from build123d import *

# Parameters (mm, degrees)
MAIN_FACE_EXTRUDE_DEPTH              = 7.4
MAIN_WALLS_EXTRUDE_DEPTH             = 35
MAIN_WALLS_LOWER_CHAMFER_SIZE        = 1
MAIN_WALLS_ENTRY_CHAMFER_SIZE        = 1
SKETCH4_W                            = 3
SKETCH4_H                            = 40.5
SERVO_MOUNT_CUT_DEPTH                = 35
SERVO_MOUNT_HOLES_REACH              = 72.134
SKETCH5_R                            = 2.25
MOUNT_DOVETAIL_DEPTH                 = 61.8
MOUNT_DOVETAIL_CHAMFER_SIZE          = 8
SKETCH9_W                            = 27.3
SKETCH9_H                            = 68.845299462
DOVETAIL_OFFSET_CUT_DEPTH            = 5
SKETCH10_R                           = 2.05
MOUNT_SCREW_HOLE_DEPTH               = 72.175838597
SKETCH11_R                           = 3.5
MOUNT_SCREW_COUNTERSINK_DEPTH        = 3
MOUNT_SCREW_COUNTERSINK_CHAMFER_SIZE = 1
GEAR_CUT_DEPTH                       = 68.031634323
GEAR_ENTRY_CHAMFER_SIZE              = 3


with BuildPart() as part:
    # Sketch1 → Main Face Extrude (new body)
    with BuildSketch(Plane(origin=(0, 0, 0), x_dir=(1, 0, 0), z_dir=(0, 1, 0))):
        Polygon((-20, 35), (7.542640687, 35), (20, 22.542640687), (20, -26.542640687), (7.542640687, -39), (-20, -39), align=None)
    extrude(amount=MAIN_FACE_EXTRUDE_DEPTH)

    # Sketch3 → Main Walls Extrude (add)
    with BuildSketch(Plane(origin=(0, 7.4, 0), x_dir=(1, 0, 0), z_dir=(0, 1, 0))):
        Polygon((-20, 35), (-20, -39), (7.542640687, -39), (20, -26.542640687), (20, 22.542640687), (7.542640687, 35), align=None)
        Polygon((-17, 32), (-17, -36), (6.3, -36), (17, -25.3), (17, 21.3), (6.3, 32), align=None, mode=Mode.SUBTRACT)
    extrude(amount=MAIN_WALLS_EXTRUDE_DEPTH)

    # Main Walls Lower Chamfer
    main_walls_lower_chamfer_edges = [part.edges().sort_by_distance(p)[0] for p in [
        (-5.35, 7.4, -32),
        (-5.35, 7.4, 36),
        (11.65, 7.4, 30.65),
        (17, 7.4, 2),
        (11.65, 7.4, -26.65),
    ]]
    chamfer(main_walls_lower_chamfer_edges, length=MAIN_WALLS_LOWER_CHAMFER_SIZE)

    # Main Walls Entry Chamfer
    main_walls_entry_chamfer_edges = [part.edges().sort_by_distance(p)[0] for p in [
        (-5.35, 42.4, -32),
        (-17, 42.4, 2),
        (-5.35, 42.4, 36),
        (11.65, 42.4, 30.65),
        (17, 42.4, 2),
        (11.65, 42.4, -26.65),
    ]]
    chamfer(main_walls_entry_chamfer_edges, length=MAIN_WALLS_ENTRY_CHAMFER_SIZE)

    # Sketch4 → Servo Mount Cut (cut)
    with BuildSketch(Plane(origin=(0, 42.4, 0), x_dir=(1, 0, 0), z_dir=(0, 1, 0))):
        with Locations((-18.5, -3.45)):
            Rectangle(SKETCH4_W, SKETCH4_H)
    extrude(amount=-SERVO_MOUNT_CUT_DEPTH, mode=Mode.SUBTRACT)

    # Sketch5 → Servo Mount Holes (cut, up to next)
    with BuildSketch(Plane.ZY.offset(20), mode=Mode.PRIVATE) as servo_mount_holes_sk1:
        with Locations((-21.6, 22.65)):
            Circle(SKETCH5_R)
    servo_mount_holes_tool1 = extrude(servo_mount_holes_sk1.sketch, amount=-SERVO_MOUNT_HOLES_REACH, mode=Mode.PRIVATE) & part.part
    # Sketch5 → Servo Mount Holes (cut, up to next)
    with BuildSketch(Plane.ZY.offset(20), mode=Mode.PRIVATE) as servo_mount_holes_sk2:
        with Locations((-21.6, 12.65)):
            Circle(SKETCH5_R)
    servo_mount_holes_tool2 = extrude(servo_mount_holes_sk2.sketch, amount=-SERVO_MOUNT_HOLES_REACH, mode=Mode.PRIVATE) & part.part
    # Sketch5 → Servo Mount Holes (cut, up to next)
    with BuildSketch(Plane.ZY.offset(20), mode=Mode.PRIVATE) as servo_mount_holes_sk3:
        with Locations((28.5, 22.65)):
            Circle(SKETCH5_R)
    servo_mount_holes_tool3 = extrude(servo_mount_holes_sk3.sketch, amount=-SERVO_MOUNT_HOLES_REACH, mode=Mode.PRIVATE) & part.part
    # Sketch5 → Servo Mount Holes (cut, up to next)
    with BuildSketch(Plane.ZY.offset(20), mode=Mode.PRIVATE) as servo_mount_holes_sk4:
        with Locations((28.5, 12.65)):
            Circle(SKETCH5_R)
    servo_mount_holes_tool4 = extrude(servo_mount_holes_sk4.sketch, amount=-SERVO_MOUNT_HOLES_REACH, mode=Mode.PRIVATE) & part.part
    add(servo_mount_holes_tool1.solids().sort_by_distance((-20, 22.65, -21.6))[0], mode=Mode.SUBTRACT)
    add(servo_mount_holes_tool2.solids().sort_by_distance((-20, 12.65, -21.6))[0], mode=Mode.SUBTRACT)
    add(servo_mount_holes_tool3.solids().sort_by_distance((-20, 22.65, 28.5))[0], mode=Mode.SUBTRACT)
    add(servo_mount_holes_tool4.solids().sort_by_distance((-20, 12.65, 28.5))[0], mode=Mode.SUBTRACT)

    # Sketch8 → Mount Dovetail (add)
    with BuildSketch(Plane.ZY.offset(20)):
        Polygon((-28.381197846, 0), (-32.422649731, -7), (-32.422649731, -8), (36.422649731, -8), (36.422649731, -7), (32.381197846, 0), align=None)
    extrude(amount=-MOUNT_DOVETAIL_DEPTH)

    # Mount Dovetail Chamfer
    mount_dovetail_chamfer_edges = [part.edges().sort_by_distance(p)[0] for p in [
        (41.8, 0, 2),
    ]]
    chamfer(mount_dovetail_chamfer_edges, length=MOUNT_DOVETAIL_CHAMFER_SIZE - 0.0001)  # a hair under: the kernel refuses the full size

    # Sketch9 → Dovetail Offset Cut (cut)
    with BuildSketch(Plane.XZ.offset(8)):
        with Locations((-6.35, 2)):
            Rectangle(SKETCH9_W, SKETCH9_H)
    extrude(amount=-DOVETAIL_OFFSET_CUT_DEPTH, mode=Mode.SUBTRACT)

    # Sketch10 → Mount Screw Hole (cut, through all)
    with BuildSketch(Plane(origin=(0, 0, 0), x_dir=(1, 0, 0), z_dir=(0, 1, 0))):
        with Locations(Location((25.8, -2, 0), (0, 0, 270))):
            Circle(SKETCH10_R)
    extrude(amount=-MOUNT_SCREW_HOLE_DEPTH, mode=Mode.SUBTRACT)

    # Sketch11 → Mount Screw Countersink (cut)
    with BuildSketch(Plane(origin=(0, 0, 0), x_dir=(1, 0, 0), z_dir=(0, 1, 0))):
        with Locations(Location((25.8, -2, 0), (0, 0, 270))):
            Circle(SKETCH11_R)
    extrude(amount=-MOUNT_SCREW_COUNTERSINK_DEPTH, mode=Mode.SUBTRACT)

    # Mount Screw Countersink Chamfer
    mount_screw_countersink_chamfer_edges = [part.edges().sort_by_distance(p)[0] for p in [
        (25.8, 0, -1.5),
    ]]
    chamfer(mount_screw_countersink_chamfer_edges, length=MOUNT_SCREW_COUNTERSINK_CHAMFER_SIZE)

    # Sketch2 → Gear Cut (cut, through all)
    with BuildSketch(Plane(origin=(0, 7.4, 0), x_dir=(1, 0, 0), z_dir=(0, 1, 0))):
        Polygon((-1.7, 26.5), (5.3, 26.5), (7.3, 24.5), (7.3, -11.5), (5.3, -13.5), (-1.7, -13.5), (-3.7, -11.5), (-3.7, 24.5), align=None)
    extrude(amount=-GEAR_CUT_DEPTH, mode=Mode.SUBTRACT)

    # Gear Entry Chamfer
    gear_entry_chamfer_edges = [part.edges().sort_by_distance(p)[0] for p in [
        (-2.7, 7.4, -25.5),
        (-3.7, 7.4, -6.5),
        (-2.7, 7.4, 12.5),
        (1.8, 7.4, 13.5),
        (6.3, 7.4, 12.5),
        (7.3, 7.4, -6.5),
        (6.3, 7.4, -25.5),
        (1.8, 7.4, -26.5),
    ]]
    chamfer(gear_entry_chamfer_edges, length=GEAR_ENTRY_CHAMFER_SIZE)


solid = part.part
The listing builds one solid part. Answer for the finished solid, in the listing's coordinates (mm). A direction names the side the tool comes from. Give positions to 0.01 mm unless a question says otherwise; leave off trailing zeros. Loops run counter-clockwise (first coordinate to the right, second up) from the corner with the lowest first, then second, coordinate; pieces in that order, holes last. Notation, with made-up numbers: (-30.75, 11.25) - (-25.75, 11.25) arc R14 cw to (-25.75, 32.25) - close; hole circle Ø11 at (41.5, 29.5). An arc over 180 degrees is marked (long way). Use one line per item in the form item = value.
1. Section D-D on x = -13 is taken. Give the vertices of the cut face in (y, z), then the cut area to 3 significant figures.
Calculated:
outline = (-3, -30.11) - (0, -28.38) - (0, -35) - (42.4, -35) - (42.4, -33) - (41.4, -32) - (8.4, -32) - (7.4, -31) - (7.4, 35) - (8.4, 36) - (41.4, 36) - (42.4, 37) - (42.4, 39) - (0, 39) - (0, 32.38) - (-3, 34.11) - close
area = 945 mm^2
2. The mould has two halves that part along X. Classify faces 1 (the face through (-19, 25, -16.8)), 2 (the face through (13.68, 20.9, 32.86)), 3 (the face through (6.3, 0.8, -25.5)): pulls with the +X half, pulls with the -X half, needs draft (parallel to the pull), parting line crosses it, or undercut.
Calculated:
face_1 = needs draft
face_2 = pulls with the +X half
face_3 = undercut
3. Section A-A on x = 25.8 is taken. Give the vertices of the cut face in (y, z).
Calculated:
outline = (-8, -32.42) - (-7, -32.42) - (0, -28.38) - (0, -2.5) - (-1, -1.5) - (-3, -1.5) - (-3, -0.05) - (-8, -0.05) - close; (-8, 4.05) - (-3, 4.05) - (-3, 5.5) - (-1, 5.5) - (0, 6.5) - (0, 32.38) - (-7, 36.42) - (-8, 36.42) - close
4. Find the intervals of material crossed by line 1 along Y through (x, z) = (-18.5, -21.6); line 2 along X through (y, z) = (-7, 2); line 3 along Y through (x, z) = (-17.85, 28.5), in increasing order. Write a range as [from, to].
Calculated:
line_1 = [-3, 10.4], [14.9, 20.4], [24.9, 42.4]
line_2 = [7.3, 23.75], [27.85, 40.8]
line_3 = [-3, 10.4], [14.9, 20.4], [24.9, 42.25]
5. Section C-C on z = 29.5 is taken. Count the separate pieces of the cut face and the enclosed holes in it, then the cut area to 3 significant figures.
Calculated:
separate_pieces = 3
enclosed_holes = 0
area = 829 mm^2
6. Which of the six approach directions +Z, -Z, +X, -X, +Y, -Y give full straight-line access (tool end or side, diameter ignored) to faces 4 (the face through (-17, 24, -25)), 5 (the face through (-10, -3, 10)), 6 (the face through (7.3, -3, 2)), 7 (the face through (-3.7, 1, -6))?
Calculated:
face_4 = +Y
face_5 = +Z, -Z, -X, -Y
face_6 = -Y
face_7 = +Y, -Y
7. Section B-B on y = 12.65 is taken. Give the vertices of the cut face in (x, z).
Calculated:
outline = (-20, -35) - (7.54, -35) - (20, -22.54) - (20, 26.54) - (7.54, 39) - (-20, 39) - (-20, 30.75) - (-17, 30.75) - (-17, 36) - (6.3, 36) - (17, 25.3) - (17, -21.3) - (6.3, -32) - (-17, -32) - (-17, -23.85) - (-20, -23.85) - close; (-20, -19.35) - (-17, -19.35) - (-17, -16.8) - (-20, -16.8) - close; (-20, 23.7) - (-17, 23.7) - (-17, 26.25) - (-20, 26.25) - close
8. Given pin 1 Ø3 at (y, z) = (32.5, -8.5) entering from +X; pin 2 Ø5.5 at (x, z) = (3, 36.5) entering from -Y; pin 3 Ø3.5 at (y, z) = (24, 31.5) entering from +X, each flat-ended and moving along its own axis, determine where each tip first touches the part or whether it passes through.
Calculated:
pin_1 = 20
pin_2 = -3
pin_3 = 16.79
